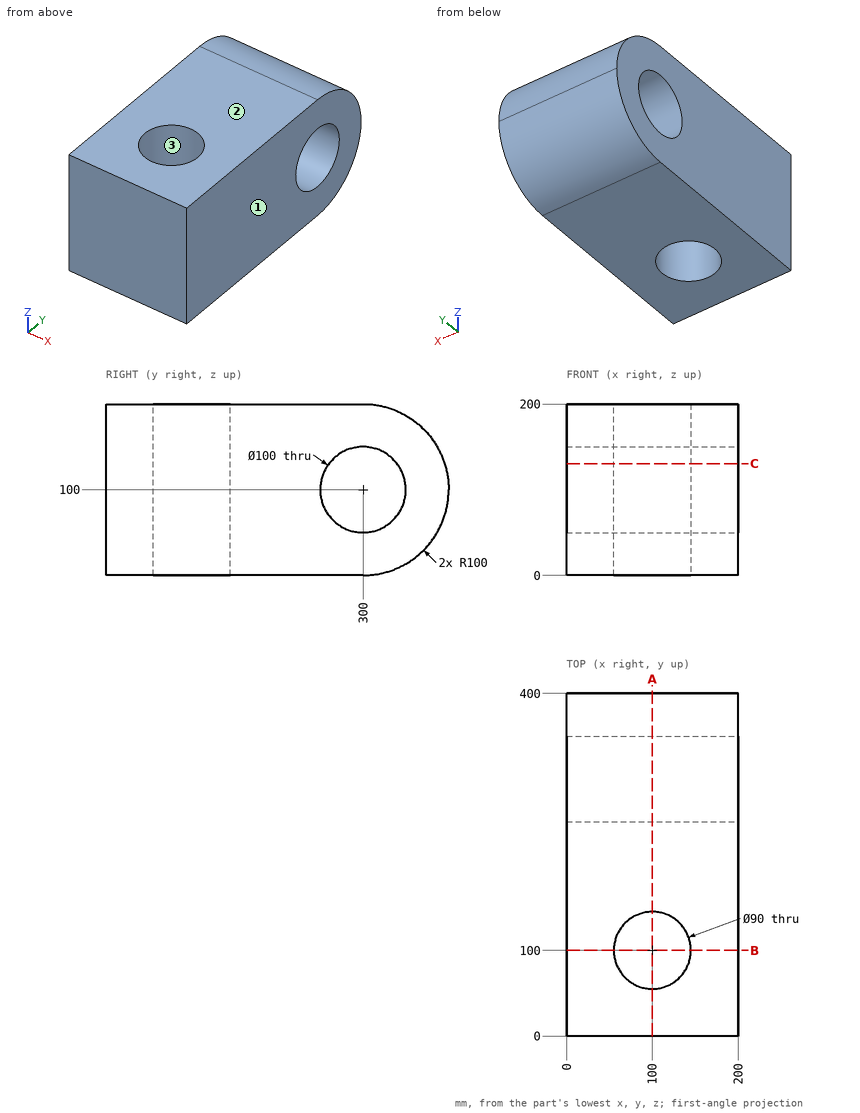
Study the drawing (mm; zero at the part's minimum x, y, z) and answer. Coordinates: 2 decimals unless noted, no trailing zeros. Loops run counter-clockwise (first coordinate to the right, second up) from the corner with the lowest first, then second, coordinate; pieces in that order, holes last. Notation, with made-up numbers: (-24, 22) -> (-2, 22) arc R19 ccw to (-2, 50) -> close; hole circle Ø6 at (50.5, 25). An arc over 180 degrees is marked (long way). Write item = value, one per line. Start each with the question number.
1) The part is cut by section C-C, the plane z = 130.5. Determine the outline of the cut face in (x, y), plus the area to 3 significant figures.
2) Given P1, Ø10, axis at x = 105.5, y = 324, coming from the +Z side, flat-ended and moving along its own axis, determine where the tip first touches the part or whether it passes through.
3) Find the intervals of material crossed by L1, parallel to Z at x = 46, y = 300; L2, parallel to Y at x = 45, z = 100; L3, parallel to X at y = 86, z = 118.5, in increasing order. Write a range as from..to.
4) The mould has two halves that part along X. Classify the marked faces 1, 2 and 3: pulls with the +X half, pulls with the -X half, needs draft (parallel to the pull), parting line crosses it, or undercut.
5) The part is cut by section B-B, the plane y = 100. Determine the outline of the cut face in (x, z), plus the area to 3 significant figures.
6) The part is cut by section A-A, the plane x = 100. State how many separate pieces and enclosed holes the cut face has, plus the area to 3 significant figures.
Result:
q1.outline = (0, 0) -> (200, 0) -> (200, 260.38) -> (0, 260.38) -> close; (0, 339.62) -> (200, 339.62) -> (200, 395.24) -> (0, 395.24) -> close; hole circle Ø90 at (100, 100)
q1.area = 56,800 mm²
q2.P1 = 198.18
q3.L1 = 0..50, 150..200
q3.L2 = 0..250, 350..400
q3.L3 = 0..57.23, 142.77..200
q4.face_1 = pulls with the +X half
q4.face_2 = needs draft
q4.face_3 = undercut
q5.outline = (0, 0) -> (55, 0) -> (55, 200) -> (0, 200) -> close; (145, 0) -> (200, 0) -> (200, 200) -> (145, 200) -> close
q5.area = 22,000 mm²
q6.separate_pieces = 2
q6.enclosed_holes = 1
q6.area = 49,900 mm²
